Geometry: final body of the model. Coordinates: model frame, mm. A direction names the side the tool comes from. Round coordinates to 2 decimals unless told otherwise and drop trailing zeros. Loops run counter-clockwise (first coordinate to the right, second up) from the corner with the lowest first, then second, coordinate; pieces in that order, holes last. Notation, with made-up numbers: (78, 3) - (99, 3) arc R13 ccw to (99, 28) - close; hole circle Ø2 at (49.25, -2.5). An arc over 180 degrees is marked (long way). Use CSV: the item, a comma, the result in double quotes.
from build123d import *

# Parameters (mm, degrees)
BOX027_W     = 9.6
BOX027_H     = 24
BOX027_DEPTH = 66.8
BOX024_W     = 11.8
BOX024_H     = 28.4
BOX024_DEPTH = 69
BOX026_W     = 17.6
BOX026_H     = 24
BOX026_DEPTH = 9.6
BOX025_W     = 17.6
BOX025_H     = 28.4
BOX025_DEPTH = 11.8


with BuildPart() as cube020:
    # Box027 → Box027 (new body)
    with BuildSketch(Plane(origin=(-9.6, 2.2, 2.2), x_dir=(1, 0, 0), z_dir=(0, 0, 1))):
        with Locations((4.8, 12)):
            Rectangle(BOX027_W, BOX027_H)
    extrude(amount=BOX027_DEPTH)


with BuildPart() as cut024:
    # Box024 → Box024 (new body)
    with BuildSketch(Plane(origin=(-11.8, 0, 0), x_dir=(1, 0, 0), z_dir=(0, 0, 1))):
        with Locations((5.9, 14.2)):
            Rectangle(BOX024_W, BOX024_H)
    extrude(amount=BOX024_DEPTH)

    # Cut024: cut Cube020
    add(cube020.part, mode=Mode.SUBTRACT)


with BuildPart() as cube019:
    # Box026 → Box026 (new body)
    with BuildSketch(Plane(origin=(0, 2.2, 2.2), x_dir=(1, 0, 0), z_dir=(0, 0, 1))):
        with Locations((8.8, 12)):
            Rectangle(BOX026_W, BOX026_H)
    extrude(amount=BOX026_DEPTH)


with BuildPart() as rohr:
    # Box025 → Box025 (new body)
    with BuildSketch(Plane.XY):
        with Locations((8.8, 14.2)):
            Rectangle(BOX025_W, BOX025_H)
    extrude(amount=BOX025_DEPTH)

    # Cut023: cut Cube019
    add(cube019.part, mode=Mode.SUBTRACT)

    # Fusion010: union Cut024
    add(cut024.part)


with BuildPart() as rohr_1:
    # Fusion010 placement: moved
    add(rohr.part.moved(Location((50.2, 32.8, 30))))


solid = rohr_1.part
Item 1: Section A-A on x = 43.75. Return the cut outline in (y, z), plus the area to 3 significant figures.
Final values:
outline,"(32.8, 30) - (61.2, 30) - (61.2, 99) - (59, 99) - (59, 32.2) - (35, 32.2) - (35, 99) - (32.8, 99) - close"
area,"356 mm²"
Item 2: Reachability of faces 5 (the flat face through (54, 47, 32.2)), 6 (the flat face through (53, 47, 30)), 7 (the flat face through (59, 60, 41.8)) from +Z, -Z, +X, -X, +Y, -Y: full face, straight path, thin tool, end or side. Return the list, or none.
Final values:
face 5,"+Z, +X"
face 6,"-Z, +X, -X, +Y, -Y"
face 7,"+Z, +X, +Y, -Y"
Item 3: Section C-C on y = 41.25. Return the cut outline in (x, z).
Final values:
outline,"(38.4, 30) - (67.8, 30) - (67.8, 32.2) - (40.6, 32.2) - (40.6, 99) - (38.4, 99) - close"
Item 4: Mould query, pull axis Y, two halves, no side actions, for faces 1 (the flat face through (46, 32.8, 56)), 2 (the flat face through (40, 47, 99)), 3 (the flat face through (48, 35, 58)), 4 (the flat face through (48, 59, 58)). Classes: released by +Y, released by -Y, zero draft, split by the parting line, or undercut.
Final values:
face 1,"released by -Y"
face 2,"zero draft"
face 3,"undercut"
face 4,"undercut"
Item 5: Section B-B on z = 64.5. Return the cut outline in (x, y), plus the area to 3 significant figures.
Final values:
outline,"(38.4, 32.8) - (50.2, 32.8) - (50.2, 35) - (40.6, 35) - (40.6, 59) - (50.2, 59) - (50.2, 61.2) - (38.4, 61.2) - close"
area,"105 mm²"
Item 6: Pin query (flat end, axial travel): P1, Ø7, axis at y = 51.5, z = 73.5, coming from the +X side; P2, Ø5, axis at x = 63, y = 43.5, coming from the +Z side; P3, Ø2.5, axis at x = 54.5, y = 60, coming from the +Z side. Return the tip coordinate at first contact, or that it passes through.
Final values:
P1,"stops at x = 40.6"
P2,"stops at z = 32.2"
P3,"stops at z = 41.8"
Item 7: Material intervals for line 1 (Y direction, x = 41, z = 42.5); line 2 (Z direction, x = 48, y = 47.75); line 3 (X direction, y = 40.5, z = 49.5), sorted ascending.
Final values:
line 1,"y = 32.8 to 35, 59 to 61.2"
line 2,"z = 30 to 32.2"
line 3,"x = 38.4 to 40.6"
